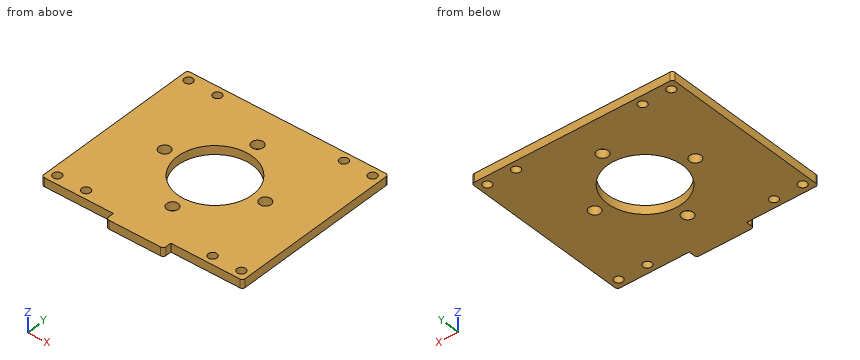
```python
from build123d import *

# Parameters (mm, degrees)
SKETCH_1_W          = 70
SKETCH_1_H          = 60
EXTRUDE_1_DEPTH     = 3
SKETCH_2_R          = 13
CUT_EXTRUDE_1_DEPTH = 47.19523785
SKETCH_3_R          = 2
CUT_EXTRUDE_2_DEPTH = 47.19523785
SKETCH_4_W          = 20
SKETCH_4_H          = 3
EXTRUDE_2_DEPTH     = 3
SKETCH_5_R          = 1.5
CUT_EXTRUDE_3_DEPTH = 49.197510309
SKETCH_6_R          = 1.5
CUT_EXTRUDE_4_DEPTH = 49.197510309
FILLET_1_R          = 1


with BuildPart() as part:
    # 草图1 → 凸台-拉伸1 (new body)
    with BuildSketch(Plane.XY):
        Rectangle(SKETCH_1_W, SKETCH_1_H)
    extrude(amount=EXTRUDE_1_DEPTH)

    # 草图2 → 切除-拉伸1 (cut, through all)
    with BuildSketch(Plane.XY.offset(3)):
        Circle(SKETCH_2_R)
    extrude(amount=-CUT_EXTRUDE_1_DEPTH, mode=Mode.SUBTRACT)

    # 草图3 → 切除-拉伸2 (cut, through all)
    with BuildSketch(Plane.XY.offset(3)):
        with Locations((0, 17.5)):
            Circle(SKETCH_3_R)
        with Locations((-17.5, 0)):
            Circle(SKETCH_3_R)
        with Locations(Location((0, -17.5, 0), (0, 0, 180))):
            Circle(SKETCH_3_R)
        with Locations(Location((17.5, 0, 0), (0, 0, 180))):
            Circle(SKETCH_3_R)
    extrude(amount=-CUT_EXTRUDE_2_DEPTH, mode=Mode.SUBTRACT)

    # 草图4 → 凸台-拉伸2 (add)
    with BuildSketch(Plane.XY.offset(3)):
        with Locations((0, -31.5)):
            Rectangle(SKETCH_4_W, SKETCH_4_H)
    extrude(amount=-EXTRUDE_2_DEPTH)

    # 草图5 → 切除-拉伸3 (cut, through all)
    with BuildSketch(Plane.XY.offset(3)):
        with Locations((-32, 27)):
            Circle(SKETCH_5_R)
        with Locations((-22, 27)):
            Circle(SKETCH_5_R)
        with Locations(Location((22, 27, 0), (0, 0, 180))):
            Circle(SKETCH_5_R)
        with Locations(Location((32, 27, 0), (0, 0, 180))):
            Circle(SKETCH_5_R)
    extrude(amount=-CUT_EXTRUDE_3_DEPTH, mode=Mode.SUBTRACT)

    # 草图6 → 切除-拉伸4 (cut, through all)
    with BuildSketch(Plane.XY.offset(3)):
        with Locations((-32, -27)):
            Circle(SKETCH_6_R)
        with Locations((-22, -27)):
            Circle(SKETCH_6_R)
        with Locations(Location((22, -27, 0), (0, 0, 180))):
            Circle(SKETCH_6_R)
        with Locations(Location((32, -27, 0), (0, 0, 180))):
            Circle(SKETCH_6_R)
    extrude(amount=-CUT_EXTRUDE_4_DEPTH, mode=Mode.SUBTRACT)

    # 圆角1
    fillet_1_edges = [part.edges().sort_by_distance(p)[0] for p in [
        (-10, -33, 1.5),
        (10, -33, 1.5),
        (35, -30, 1.5),
        (-35, -30, 1.5),
        (-35, 30, 1.5),
        (35, 30, 1.5),
    ]]
    fillet(fillet_1_edges, radius=FILLET_1_R)


solid = part.part
```
Input: part model. Units: mm. Frame: model coordinates. Give positions to 0.01 mm unless a question says otherwise; leave off trailing zeros. Write each loop counter-clockwise with the first axis right and the second up, starting at its lowest first coordinate (ties: lowest second). Pieces come first, ordered by that corner, then holes. Notation, with made-up numbers: (-0.75, -6.75) - (32.25, -6.75) arc R35 cw to (32.25, 32.25) - close; hole circle Ø5 at (22.25, 27.25). An arc over 180 degrees is marked (long way). Write item = value, one per line. Start each with the question number.
1) Cut plane B-B (x = 17.5). Return loops of the section in (y, z).
2) Material intervals for L1, parallel to Y at x = -22, z = 2.2; L2, parallel to Y at x = -1, z = 2.3; L3, parallel to Y at x = -0.5, z = 2.2, sorted ascending. Write a range as [from, to].
3) Cut plane C-C (z = 2.1). Give the number of separate pieces and of enclosed holes in the cut face, and give its area (3 significant figures).
4) Pin query (flat end, axial travel): pin 1 (1 mm diameter, centred on x = 28, z = 2.5, fed in from -Y); pin 2 (0.6 mm diameter, centred on y = -30.5, z = 2, fed in from -X). Return the tip coordinate at first contact, or that it passes through.
5) Cut plane A-A (y = -27). Return loops of the section in (x, z).
6) Cut plane D-D (x = 0). Return loops of the section in (y, z), and give its area (3 significant figures).
Answers follow:
q1.outline = (-30, 0) - (-2, 0) - (-2, 3) - (-30, 3) - close; (2, 0) - (30, 0) - (30, 3) - (2, 3) - close
q2.L1 = [-30, -28.5], [-25.5, 25.5], [28.5, 30]
q2.L2 = [-33, -19.23], [-15.77, -12.96], [12.96, 15.77], [19.23, 30]
q2.L3 = [-33, -19.44], [-15.56, -12.99], [12.99, 15.56], [19.44, 30]
q3.separate_pieces = 1
q3.enclosed_holes = 13
q3.area = 3,620 mm^2
q4.pin_1 = -30
q4.pin_2 = -10
q5.outline = (-35, 0) - (-33.5, 0) - (-33.5, 3) - (-35, 3) - close; (-30.5, 0) - (-23.5, 0) - (-23.5, 3) - (-30.5, 3) - close; (-20.5, 0) - (20.5, 0) - (20.5, 3) - (-20.5, 3) - close; (23.5, 0) - (30.5, 0) - (30.5, 3) - (23.5, 3) - close; (33.5, 0) - (35, 0) - (35, 3) - (33.5, 3) - close
q6.outline = (-33, 0) - (-19.5, 0) - (-19.5, 3) - (-33, 3) - close; (-15.5, 0) - (-13, 0) - (-13, 3) - (-15.5, 3) - close; (13, 0) - (15.5, 0) - (15.5, 3) - (13, 3) - close; (19.5, 0) - (30, 0) - (30, 3) - (19.5, 3) - close
q6.area = 87.0 mm^2
